Source: three-view drawing plus pictorial views. Frame: mm from the lowest corner of the part. Give positions to 0.01 mm unless a question says otherwise; leave off trailing zeros. Order: outer loops, then holes, each group sorted by start corner. A loop starts at its lowest first (then second) coordinate and runs counter-clockwise, first axis right, second up. Notation, with made-up numbers: (75, -30.5) -> (109, -30.5) arc R14 ccw to (109, -5.5) -> close; hole circle Ø6 at (27.25, -36). An arc over 180 degrees is marked (long way). Answer in a Markdown table with one row per item.
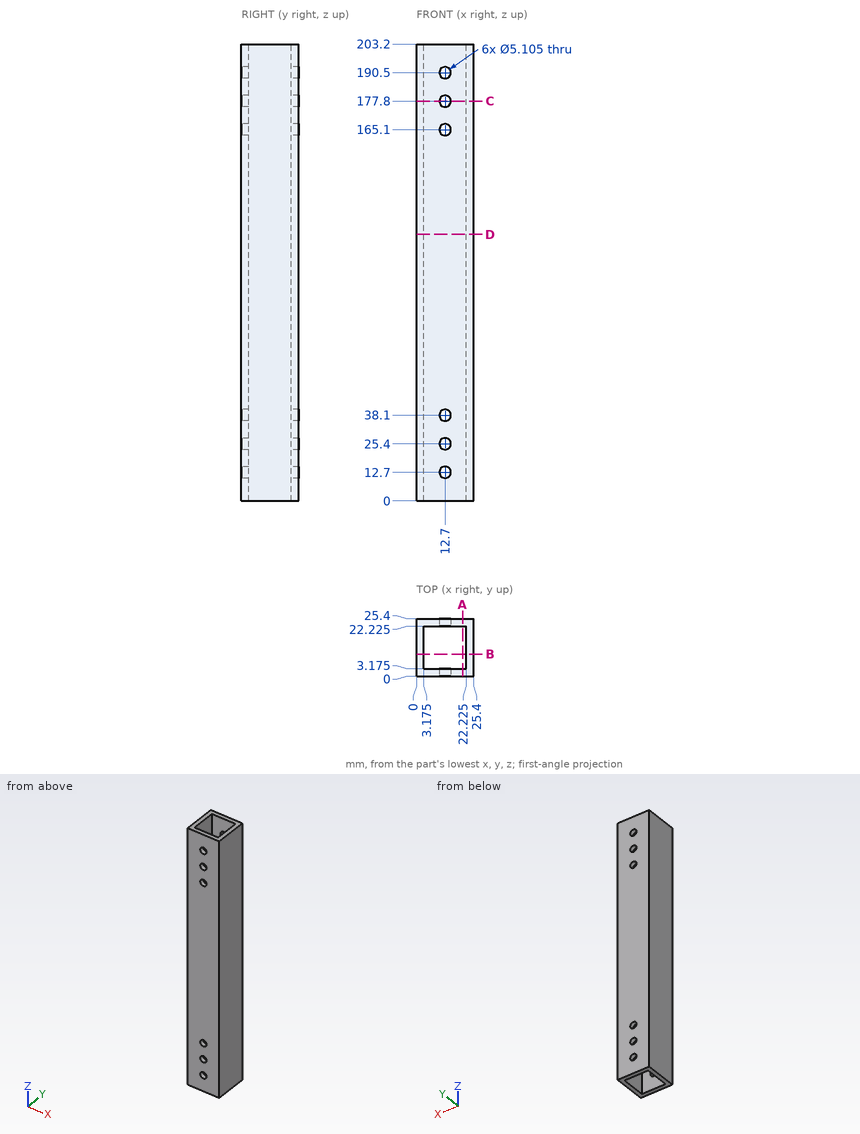
(1) Ray query, probe 1 along X at (y, z) = (23.75, 190.5); probe 2 along X at (y, z) = (19, 68) (1 decimal). Return the intervals inside material, ascending.
A:
| item | result |
|---|---|
| probe 1 | x = 0 to 10.15, 15.25 to 25.4 |
| probe 2 | x = 0 to 3.2, 22.2 to 25.4 |
(2) Section query D-D (z = 118.5). Return the cut outline in (x, y) (1 decimal), plus the area to 3 significant figures.
A:
| item | result |
|---|---|
| outline | (0, 0) -> (25.4, 0) -> (25.4, 25.4) -> (0, 25.4) -> close; hole (3.2, 3.2) -> (22.2, 3.2) -> (22.2, 22.2) -> (3.2, 22.2) -> close |
| area | 282 mm^2 |
(3) Section query A-A (x = 20.5). Return the cut outline in (y, z) (1 decimal).
A:
| item | result |
|---|---|
| outline | (0, 0) -> (3.2, 0) -> (3.2, 203.2) -> (0, 203.2) -> close; (22.2, 0) -> (25.4, 0) -> (25.4, 203.2) -> (22.2, 203.2) -> close |
(4) First-contact query: pin 1 Ø3 at (x, z) = (12.7, 177.8) entering from -Y. Flat tip, straight axial feed; report the tip coordinate or a pass-through.
A:
| item | result |
|---|---|
| pin 1 | passes through |
(5) Section query C-C (z = 177.8). Return the cut outline in (x, y) (1 decimal).
A:
| item | result |
|---|---|
| outline | (0, 0) -> (10.1, 0) -> (10.1, 3.2) -> (3.2, 3.2) -> (3.2, 22.2) -> (10.1, 22.2) -> (10.1, 25.4) -> (0, 25.4) -> close; (15.3, 0) -> (25.4, 0) -> (25.4, 25.4) -> (15.3, 25.4) -> (15.3, 22.2) -> (22.2, 22.2) -> (22.2, 3.2) -> (15.3, 3.2) -> close |
